Read the model definition and answer for the solid it produces. Units are mm, in the model's axes. A direction names the side the tool comes from. Coordinates: 2 decimals unless noted, no trailing zeros. Write each loop counter-clockwise with the first axis right and the second up, starting at its lowest first coordinate (ties: lowest second). Pieces come first, ordered by that corner, then holes. Notation, with made-up numbers: (4, 42.25) -> (45, 42.25) arc R14 cw to (45, 69.25) -> close; hole circle Ø3 at (17.5, 68). An arc over 180 degrees is marked (long way). Answer in a Markdown table with one row per item. Add a question column.
Item 1: Straight lines are drawn through the part: line 1 (Z direction, x = 24.5, y = 6.5); line 2 (Z direction, x = 10.5, y = -27); line 3 (X direction, y = -31, z = -114). For each, find the intervals that lie inside material, in ascending order. Write a range as from..to.
Item 2: Section A-A on y = -7.88 is taken. Count the separate pieces of the cut face and the enclosed holes in it, then the cut area to 3 significant figures.
Item 3: For a pull along Y with two mould halves and no side action, classify faces 6 (the face through (9, 43, 4.6)), 7 (the face through (39, -24, 0)) as +Y half, -Y half, draft (parallel to the pull), parting line (faces both ways), or undercut.
Item 4: Section C-C on z = -26.5 is taken. Write down the section's boundary in (x, y).
Item 5: Which of the six approach directions +Z, -Z, +X, -X, +Y, -Y give full straight-line access (tool end or side, diameter ignored) to faces 1 (the face through (20.646, -34.059, -112.886)), 2 (the face through (36.97, -21.41, 2.27)), 3 (the face through (1, -1, -124.916)), 4 (the face through (-34.059, 20.646, -89.489)), 5 (the face through (34.53, 20.646, -153.402))?
Item 6: Section D-D on z = -58.5 is taken. Write down the section's boundary in (x, y).
Item 7: Given pin 1 Ø10.5 at (x, y) = (23.64, -39.4) entering from -Z; pin 2 Ø2 at (x, y) = (9, -40) entering from +Z; pin 3 Ø10.5 at (x, y) = (39.4, -7.88) entering from -Z; pin 4 Ø3 at (x, y) = (15.5, -4.5) entering from +Z, each flat-ended and moving along its own axis, determine where each tip first touches the part or whether it passes through.
```python
from build123d import *

# Parameters (mm, degrees)
F0_W      = 94.8
F0_H      = 94.8
F0_W_2    = 50.8
F0_H_2    = 50.8
F1_DEPTH  = 165.1
F2_DEPTH  = 12.7
F4_DEPTH  = 101.3
F6_DEPTH  = 114
F8_DEPTH  = 110
F9_DEPTH  = 114
F11_DEPTH = 115
F12_R     = 4.7
F12_R_2   = 3.3
F13_DEPTH = 4.6


with BuildPart() as f1:
    # F0 (on Top) → F1 (new body)
    with BuildSketch(Plane.XY):
        Rectangle(F0_W, F0_H)
        Rectangle(F0_W_2, F0_H_2, mode=Mode.SUBTRACT)
        Rectangle(F0_W_2, F0_H_2)
    extrude(amount=-F1_DEPTH)

    # F0 (on Top) → F2 (cut)
    with BuildSketch(Plane.XY):
        Rectangle(F0_W_2, F0_H_2)
    extrude(amount=-F2_DEPTH, mode=Mode.SUBTRACT)

    # F3 (on face) → F4 (cut)
    with BuildSketch(Plane.YZ.offset(47.4)):
        Polygon((0, -141.370904), (-13.7, -141.370904), (-27.4, -165.1), (-13.7, -188.829096), (13.7, -188.829096), (27.4, -165.1), (13.7, -141.370904), align=None)
    extrude(amount=-F4_DEPTH, mode=Mode.SUBTRACT)

    # F5 (on face) → F6 (cut)
    with BuildSketch(Plane.XZ.offset(47.4)):
        Polygon((13.7, -141.370904), (-13.7, -141.370904), (-27.4, -165.1), (27.4, -165.1), align=None)
    extrude(amount=-F6_DEPTH, mode=Mode.SUBTRACT)

    # F7 (on face) → F8 (cut)
    with BuildSketch(Plane(origin=(0, 47.4, 0), x_dir=(-1, 0, 0), z_dir=(0, 1, 0))):
        Polygon((13.7, -20), (-13.7, -20), (-27.4, -43.729096), (-13.7, -67.458192), (13.7, -67.458192), (27.4, -43.729096), align=None)
    extrude(amount=-F8_DEPTH, mode=Mode.SUBTRACT)

    # F7 (on face) → F9 (cut)
    with BuildSketch(Plane(origin=(0, 47.4, 0), x_dir=(-1, 0, 0), z_dir=(0, 1, 0))):
        Polygon((13.7, -77.458192), (-13.7, -77.458192), (-27.4, -101.187288), (-13.7, -124.916384), (13.7, -124.916384), (27.4, -101.187288), align=None)
    extrude(amount=-F9_DEPTH, mode=Mode.SUBTRACT)

    # F10 (on face) → F11 (cut)
    with BuildSketch(Plane.YZ.offset(47.4)):
        Polygon((13.7, -20), (-13.7, -20), (-27.4, -43.729096), (-13.7, -67.458192), (13.7, -67.458192), (27.4, -43.729096), align=None)
        Polygon((13.7, -77.458192), (-13.7, -77.458192), (-27.4, -101.187288), (-13.7, -124.916384), (13.7, -124.916384), (27.4, -101.187288), align=None)
    extrude(amount=-F11_DEPTH, mode=Mode.SUBTRACT)

    # F12 (on face) → F13 (join)
    with BuildSketch(Plane.XY):
        with Locations((-39.4, 39.4)):
            Circle(F12_R)
        with Locations((-39.4, 39.4)):
            Circle(F12_R_2, mode=Mode.SUBTRACT)
        with Locations((-39.4, 23.64)):
            Circle(F12_R)
        with Locations((-39.4, 23.64)):
            Circle(F12_R_2, mode=Mode.SUBTRACT)
        with Locations((-39.4, 7.88)):
            Circle(F12_R)
        with Locations((-39.4, 7.88)):
            Circle(F12_R_2, mode=Mode.SUBTRACT)
        with Locations((-39.4, -7.88)):
            Circle(F12_R)
        with Locations((-39.4, -7.88)):
            Circle(F12_R_2, mode=Mode.SUBTRACT)
        with Locations((-39.4, -23.64)):
            Circle(F12_R)
        with Locations((-39.4, -23.64)):
            Circle(F12_R_2, mode=Mode.SUBTRACT)
        with Locations((-39.4, -39.4)):
            Circle(F12_R)
        with Locations((-39.4, -39.4)):
            Circle(F12_R_2, mode=Mode.SUBTRACT)
        with Locations((-23.64, -39.4)):
            Circle(F12_R)
        with Locations((-23.64, -39.4)):
            Circle(F12_R_2, mode=Mode.SUBTRACT)
        with Locations((-7.88, -39.4)):
            Circle(F12_R)
        with Locations((-7.88, -39.4)):
            Circle(F12_R_2, mode=Mode.SUBTRACT)
        with Locations((-23.64, 39.4)):
            Circle(F12_R)
        with Locations((-23.64, 39.4)):
            Circle(F12_R_2, mode=Mode.SUBTRACT)
        with Locations((-7.88, 39.4)):
            Circle(F12_R)
        with Locations((-7.88, 39.4)):
            Circle(F12_R_2, mode=Mode.SUBTRACT)
        with Locations((7.88, 39.4)):
            Circle(F12_R)
        with Locations((7.88, 39.4)):
            Circle(F12_R_2, mode=Mode.SUBTRACT)
        with Locations((23.64, 39.4)):
            Circle(F12_R)
        with Locations((23.64, 39.4)):
            Circle(F12_R_2, mode=Mode.SUBTRACT)
        with Locations((39.4, 39.4)):
            Circle(F12_R)
        with Locations((39.4, 39.4)):
            Circle(F12_R_2, mode=Mode.SUBTRACT)
        with Locations((39.4, 23.64)):
            Circle(F12_R)
        with Locations((39.4, 23.64)):
            Circle(F12_R_2, mode=Mode.SUBTRACT)
        with Locations((39.4, 7.88)):
            Circle(F12_R)
        with Locations((39.4, 7.88)):
            Circle(F12_R_2, mode=Mode.SUBTRACT)
        with Locations((39.4, -7.88)):
            Circle(F12_R)
        with Locations((39.4, -7.88)):
            Circle(F12_R_2, mode=Mode.SUBTRACT)
        with Locations((39.4, -23.64)):
            Circle(F12_R)
        with Locations((39.4, -23.64)):
            Circle(F12_R_2, mode=Mode.SUBTRACT)
        with Locations((39.4, -39.4)):
            Circle(F12_R)
        with Locations((39.4, -39.4)):
            Circle(F12_R_2, mode=Mode.SUBTRACT)
        with Locations((23.64, -39.4)):
            Circle(F12_R)
        with Locations((23.64, -39.4)):
            Circle(F12_R_2, mode=Mode.SUBTRACT)
        with Locations((7.88, -39.4)):
            Circle(F12_R)
        with Locations((7.88, -39.4)):
            Circle(F12_R_2, mode=Mode.SUBTRACT)
    extrude(amount=F13_DEPTH)


solid = f1.part
```
Results below:
| question | item | result |
|---|---|---|
| 1 | line 1 | z = -141.37..-124.92, -77.46..-67.46, -20..-12.7 |
| 1 | line 2 | z = -141.37..-124.92, -77.46..-67.46, -20..0 |
| 1 | line 3 | x = -47.4..-20, 20..47.4 |
| 2 | separate pieces | 3 |
| 2 | enclosed holes | 0 |
| 2 | area | 3,780 mm2 |
| 3 | face 6 | draft |
| 3 | face 7 | undercut |
| 4 | outline | (-47.4, -47.4) -> (-17.45, -47.4) -> (-17.45, -17.45) -> (-47.4, -17.45) -> close; (-47.4, 17.45) -> (-17.45, 17.45) -> (-17.45, 47.4) -> (-47.4, 47.4) -> close; (17.45, -47.4) -> (47.4, -47.4) -> (47.4, -17.45) -> (17.45, -17.45) -> close; (17.45, 17.45) -> (47.4, 17.45) -> (47.4, 47.4) -> (17.45, 47.4) -> close |
| 5 | face 1 | +Y, -Y |
| 5 | face 2 | +Z |
| 5 | face 3 | none |
| 5 | face 4 | +X, -X |
| 5 | face 5 | -Z, +X, -X |
| 6 | outline | (-47.4, -47.4) -> (-18.87, -47.4) -> (-18.87, -18.87) -> (-47.4, -18.87) -> close; (-47.4, 18.87) -> (-18.87, 18.87) -> (-18.87, 47.4) -> (-47.4, 47.4) -> close; (18.87, -47.4) -> (47.4, -47.4) -> (47.4, -18.87) -> (18.87, -18.87) -> close; (18.87, 18.87) -> (47.4, 18.87) -> (47.4, 47.4) -> (18.87, 47.4) -> close |
| 7 | pin 1 | stops at z = -165.1 |
| 7 | pin 2 | stops at z = 0 |
| 7 | pin 3 | stops at z = -141.37 |
| 7 | pin 4 | stops at z = -12.7 |
